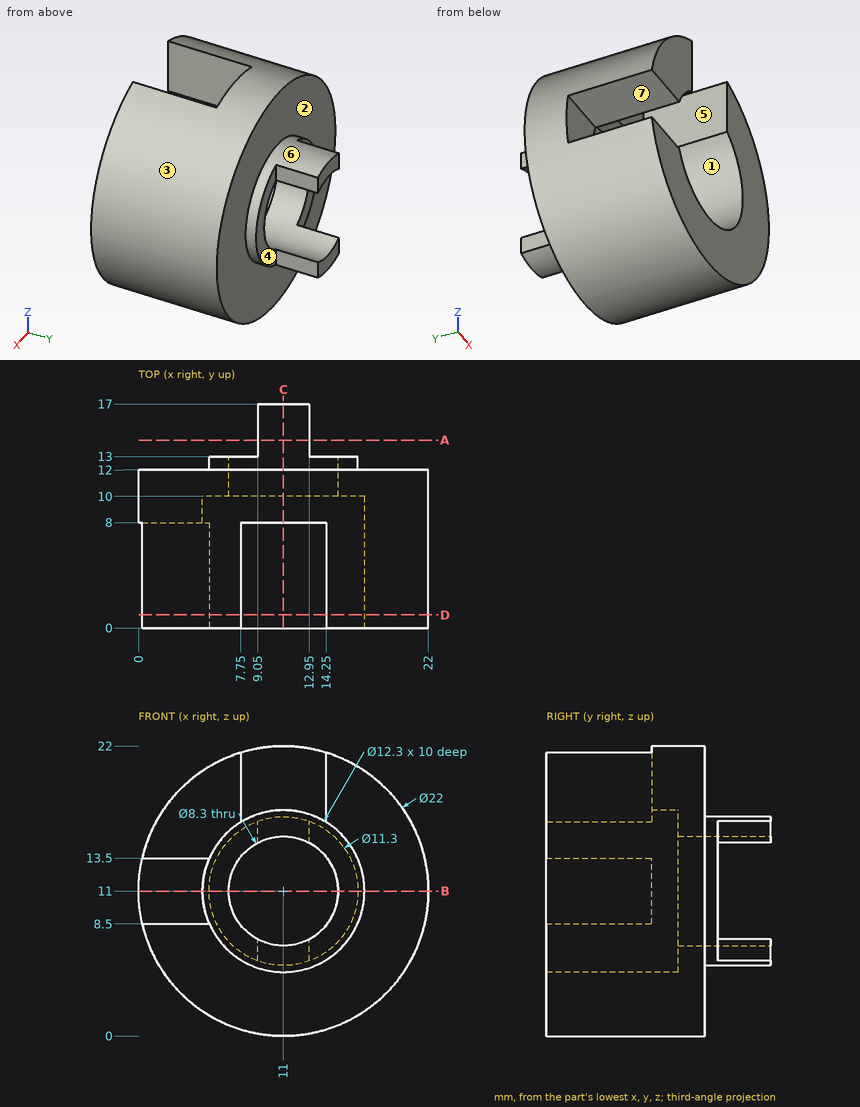
Geometry: see drawing. Coordinates: mm, zero at the bounding-box minimum. A direction names the side the tool comes from. Give positions to 0.01 mm unless a question says otherwise; leave off trailing zeros. Loops run counter-clockwise (first coordinate to the right, second up) from the corner with the lowest first, then second, coordinate; pieces in that order, holes last. Notation, with made-up numbers: M 61,-30 L 98,-30 A16 cw 98,-3 Z; hole C 73,80.5 d6. An arc over 180 degrees is marked long. Use one line per item in the form item = value.
1. Pull-direction query (Z, two-part tool) for the marked faces 1, 2 and 3; classes: released by +Z, released by -Z, zero draft, split by the parting line, or undercut.
Numbers:
face_1 = undercut
face_2 = zero draft
face_3 = split by the parting line
2. Section query A-A, the plane y = 14.25. Return the cut outline in (x, z).
Numbers:
outline = M 9.05,5.7 A5.65 ccw 12.95,5.7 L 12.95,7.34 A4.15 cw 9.05,7.34 Z; M 9.05,14.66 A4.15 cw 12.95,14.66 L 12.95,16.3 A5.65 ccw 9.05,16.3 Z
3. Section query B-B, the plane z = 11. Return the cut outline in (x, y), and give its area (3 significant figures).
Numbers:
outline = M 0,8 L 4.85,8 L 4.85,10 L 6.85,10 L 6.85,13 L 5.35,13 L 5.35,12 L 0,12 Z; M 15.15,10 L 17.15,10 L 17.15,0 L 22,0 L 22,12 L 16.65,12 L 16.65,13 L 15.15,13 Z
area = 88.6 mm²
4. Section query C-C, the plane x = 11. Return the cut outline in (y, z), and give its area (3 significant figures).
Numbers:
outline = M 0,0 L 12,0 L 12,5.35 L 17,5.35 L 17,6.85 L 10,6.85 L 10,4.85 L 0,4.85 Z; M 8,17.15 L 10,17.15 L 10,15.15 L 17,15.15 L 17,16.65 L 12,16.65 L 12,22 L 8,22 Z
area = 101 mm²
5. Reachability of the marked faces 4, 5, 6 and 7 from +Z, -Z, +X, -X, +Y, -Y: full face, straight path, thin tool, end or side. Return the list, or none.
Numbers:
face_4 = +Z, -Z, +X, +Y
face_5 = +Z, -Y
face_6 = +Y
face_7 = -X, -Y
6. First-contact query: pin 1 (10 mm diameter, centred on x = 15.5, z = 11, fed in from +Y); pin 2 (1.1 mm diameter, centred on x = 8, z = 13.5, fed in from +Y); pin 3 (1.5 mm diameter, centred on x = 3.5, z = 10.5, fed in from -Y); pin 4 (10 mm diameter, centred on y = 7.5, z = 18, fed in from +X). Flat tips, straight axial feed; report the tip coordinate or a pass-through.
Numbers:
pin_1 = 17
pin_2 = 13
pin_3 = 8
pin_4 = 21.82
7. Section query D-D, the plane y = 1. Return the cut outline in (x, z), and give its area (3 significant figures).
Numbers:
outline = M 0.29,8.5 A11 ccw long 14.25,21.51 L 14.25,16.22 A6.15 cw long 5.38,8.5 Z; M 0.29,13.5 L 5.38,13.5 A6.15 cw 7.75,16.22 L 7.75,21.51 A11 ccw Z
area = 204 mm²
8. Line query: L1, parallel to Z at x = 11, y = 15; L2, parallel to Y at x = 4.75, z = 15.5; L3, parallel to Z at x = 7, y = 9. Output: solid intervals per line, ascending.
Numbers:
L1 = 5.35 to 6.85, 15.15 to 16.65
L2 = 0 to 12
L3 = 0.75 to 6.33, 15.67 to 21.25
